Design review of the part built by this model. Coordinates are the model's own, in mm. Face numbers are marked on the shaded views. Give positions to 0.01 mm unless a question says otherwise; leave off trailing zeros. Write each loop counter-clockwise with the first axis right and the second up, starting at its lowest first coordinate (ties: lowest second). Pieces come first, ordered by that corner, then holes. Notation, with made-up numbers: M -24,-12.75 L 1,-12.75 A13 ccw 1,-5.75 Z; hole C -21,1.5 d1. An arc over 180 degrees is marked long. Use a Markdown table: item, result. Add a question column.
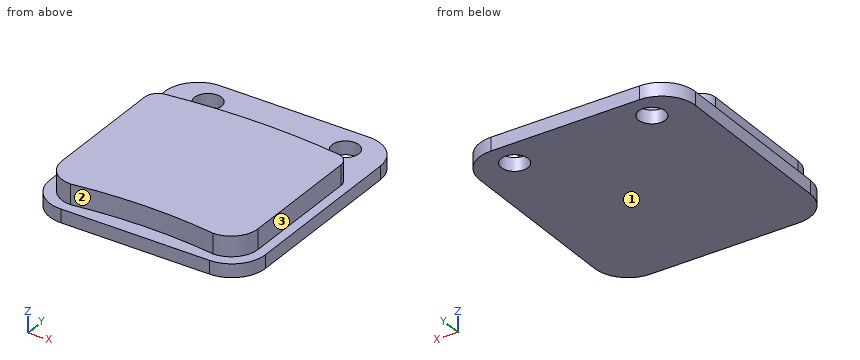
```python
from build123d import *

# Parameters (mm, degrees)
SKETCH1_R           = 2.54
BOSS_EXTRUDE1_DEPTH = 2.54
BOSS_EXTRUDE2_DEPTH = 3.81


with BuildPart() as part:
    # Sketch1 → Boss-Extrude1 (new body)
    with BuildSketch(Plane.XY):
        with BuildLine():
            Line((-14.097, -22.606), (14.097, -22.606))
            ThreePointArc((14.097, -22.606), (18.587128061, -20.746128061), (20.447, -16.256))
            Line((20.447, -16.256), (20.447, 16.256))
            ThreePointArc((20.447, 16.256), (18.587128061, 20.746128061), (14.097, 22.606))
            Line((14.097, 22.606), (-14.097, 22.606))
            ThreePointArc((-14.097, 22.606), (-18.587128061, 20.746128061), (-20.447, 16.256))
            Line((-20.447, 16.256), (-20.447, -16.256))
            ThreePointArc((-20.447, -16.256), (-18.587128061, -20.746128061), (-14.097, -22.606))
        make_face()
        with Locations((13.0175, 17.481804688)):
            Circle(SKETCH1_R, mode=Mode.SUBTRACT)
        with Locations((-13.0175, 17.481804688)):
            Circle(SKETCH1_R, mode=Mode.SUBTRACT)
    extrude(amount=BOSS_EXTRUDE1_DEPTH)

    # Sketch2 → Boss-Extrude2 (add)
    with BuildSketch(Plane.XY.offset(2.54)):
        with BuildLine():
            Line((-18.603310345, -15.583823179), (-18.603310345, 7.849049019))
            ThreePointArc((-18.603310345, 7.849049019), (-17.97174813, 9.525194962), (-16.391133005, 10.367805121))
            ThreePointArc((-16.391133005, 10.367805121), (0, 11.43), (16.391133005, 10.367805121))
            ThreePointArc((16.391133005, 10.367805121), (17.97174813, 9.525194962), (18.603310345, 7.849049019))
            Line((18.603310345, 7.849049019), (18.603310345, -15.583823179))
            ThreePointArc((18.603310345, -15.583823179), (17.094874343, -19.189362325), (13.472365536, -20.656577934))
            ThreePointArc((13.472365536, -20.656577934), (-0.025728715, -19.705190714), (-13.523310345, -20.663823179))
            ThreePointArc((-13.523310345, -20.663823179), (-17.115412793, -19.175925628), (-18.603310345, -15.583823179))
        make_face()
    extrude(amount=BOSS_EXTRUDE2_DEPTH)


solid = part.part
```
(1) Wall thickness on L1, parallel to X at y = 16, z = 0.75; L2, parallel to Y at x = -13, z = 1.5; L3, parallel to Z at x = 7, y = 20: over which ranges is each line inside the solid? List them lowest first.
(2) Add section A-A on x = -11.5. Give the boundary of the cut face in (y, z).
(3) For pin 1 (6 mm diameter, centred on x = 13.02, y = 17.48, fed in from +Z); pin 2 (1 mm diameter, centred on x = -0.5, z = 5, fed in from +Y); pin 3 (1.1 mm diameter, centred on y = 1, z = 5.5, fed in from +X), all flat-tipped, find the tip position at first contact; note any pin that passes through.
(4) Add section C-C on y = -8. Give the boundary of the cut face in (x, z), then the cut area to 3 significant figures.
(5) The part is to be moulded in two halves that separate along X. For the marked faces 1, 2 and 3, say which applies: released by +X, released by -X, zero draft, split by the parting line, or undercut.
(6) Add section D-D on x = -3.5. Give the boundary of the cut face in (y, z).
(7) Add section B-B on z = 1.75. Give the boundary of the cut face in (x, y).
From the geometry:
| question | item | result |
|---|---|---|
| 1 | L1 | x = -20.45 to -15.08, -10.95 to 10.95, 15.08 to 20.45 |
| 1 | L2 | y = -22.61 to 14.94, 20.02 to 22.61 |
| 1 | L3 | z = 0 to 2.54 |
| 2 | outline | M -22.61,0 L 15.44,0 L 15.44,2.54 L 10.91,2.54 L 10.91,6.35 L -20.4,6.35 L -20.4,2.54 L -22.61,2.54 Z; M 19.52,0 L 22.61,0 L 22.61,2.54 L 19.52,2.54 Z |
| 3 | pin 1 | stops at z = 2.54 |
| 3 | pin 2 | stops at y = 11.43 |
| 3 | pin 3 | stops at x = 18.6 |
| 4 | outline | M -20.45,0 L 20.45,0 L 20.45,2.54 L 18.6,2.54 L 18.6,6.35 L -18.6,6.35 L -18.6,2.54 L -20.45,2.54 Z |
| 4 | area | 246 mm^2 |
| 5 | face 1 | zero draft |
| 5 | face 2 | undercut |
| 5 | face 3 | released by +X |
| 6 | outline | M -22.61,0 L 22.61,0 L 22.61,2.54 L 11.38,2.54 L 11.38,6.35 L -19.77,6.35 L -19.77,2.54 L -22.61,2.54 Z |
| 7 | outline | M -20.45,-16.26 A6.35 ccw -14.1,-22.61 L 14.1,-22.61 A6.35 ccw 20.45,-16.26 L 20.45,16.26 A6.35 ccw 14.1,22.61 L -14.1,22.61 A6.35 ccw -20.45,16.26 Z; hole C -13.02,17.48 d5.08; hole C 13.02,17.48 d5.08 |
